Study the drawing (mm; zero at the part's minimum x, y, z) and answer. A direction names the side the tool comes from. Round coordinates to 2 decimals unless told otherwise and drop trailing zeros. Write each loop counter-clockwise with the first axis right and the second up, starting at its lowest first coordinate (ties: lowest second). Pieces come first, ordered by that corner, then holes. Notation, with made-up numbers: (17.25, 43.25) -> (51.25, 43.25) arc R19 cw to (51.25, 76.25) -> close; hole circle Ø7 at (71.25, 63.25). An arc over 180 degrees is marked (long way). Return JSON: item names as keys, results as strings.
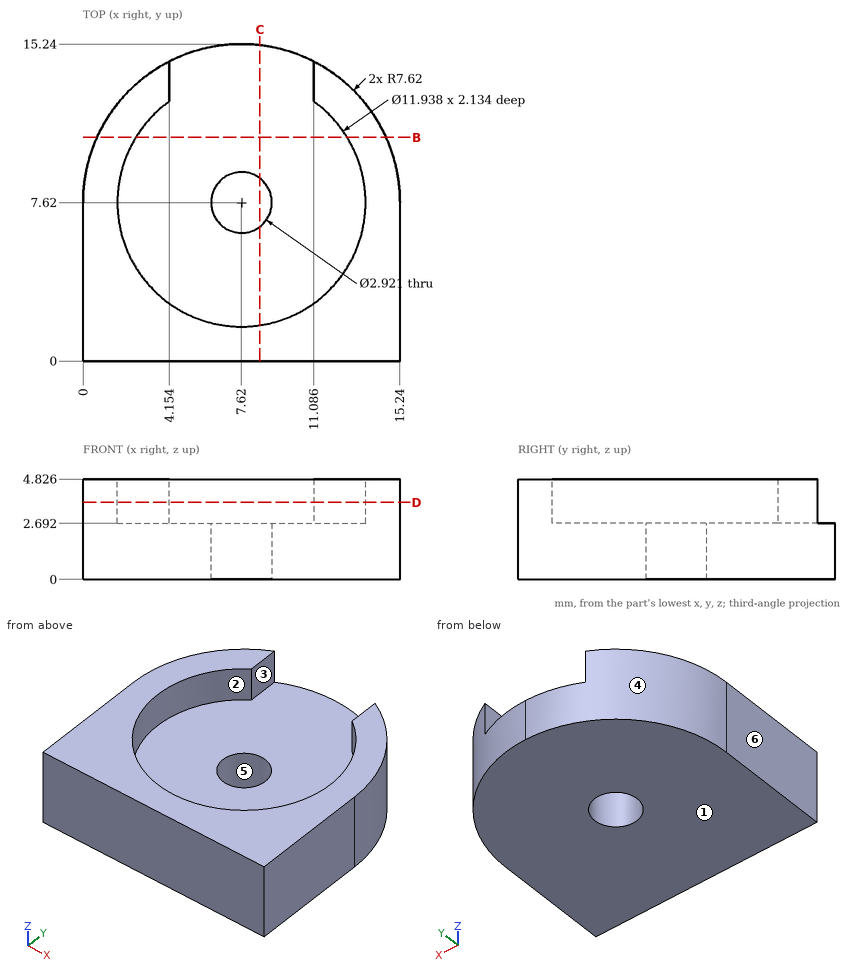
Item 1: Section B-B (y = 10.75) is taken. Give the vertices of the cut face in (x, z).
Worked answers:
{"outline": "(0.67, 0) -> (14.57, 0) -> (14.57, 4.83) -> (12.7, 4.83) -> (12.7, 2.69) -> (2.54, 2.69) -> (2.54, 4.83) -> (0.67, 4.83) -> close"}
Item 2: Flat-ended cylindrical pins translate along their axes: pin 1 (4 mm diameter, centred on x = 7.62, y = 7.62, fed in from -Z); pin 2 (1 mm diameter, centred on y = 13.5, z = 4, fed in from +X) (1 decimal); pin 3 (0.6 mm diameter, centred on y = 13.5, z = 3.5, fed in from -X). Find the tip coordinate at first contact, or state that the pin passes through.
Worked answers:
{"pin 1": "stops at z = 0", "pin 2": "stops at x = 13", "pin 3": "stops at x = 2.43"}
Item 3: For a pull along Y with two mould halves and no side action, classify the marked faces 4, 5 and 6 as released by +Y, released by -Y, zero draft, split by the parting line, or undercut.
Worked answers:
{"face 4": "released by +Y", "face 5": "undercut", "face 6": "zero draft"}
Item 4: A tool of negligible diameter and unlimited length cuts with its end or side. For the marked faces 1, 2 and 3, from which of +Z, -Z, +X, -X, +Y, -Y can it reach the whole face along a straight path? Write none if from no direction.
Worked answers:
{"face 1": "-Z, +X, -X, +Y, -Y", "face 2": "+Z", "face 3": "+Z, +Y"}
Item 5: Straight lines are drawn through the part: L1, parallel to Y at x = 7.62, z = 2.15; L2, parallel to X at y = 7.62, z = 4.05; L3, parallel to Z at x = 8, y = 13.5. For each, find the intervals that lie inside material, in ascending order. Write a range as [from, to].
Worked answers:
{"L1": "y = [0, 6.16], [9.08, 15.24]", "L2": "x = [0, 1.65], [13.59, 15.24]", "L3": "z = [0, 2.69]"}
Item 6: Section C-C (x = 8.5) is taken. Give the vertices of the cut face in (y, z) (1 decimal).
Worked answers:
{"outline": "(0, 0) -> (6.5, 0) -> (6.5, 2.7) -> (1.7, 2.7) -> (1.7, 4.8) -> (0, 4.8) -> close; (8.8, 0) -> (15.2, 0) -> (15.2, 2.7) -> (8.8, 2.7) -> close"}
Item 7: Section D-D (z = 3.7) is taken. Give the vertices of the cut face in (x, y) (1 decimal).
Worked answers:
{"outline": "(0, 0) -> (15.2, 0) -> (15.2, 7.6) arc R7.6 ccw to (11.1, 14.4) -> (11.1, 12.5) arc R6 cw (long way) to (4.2, 12.5) -> (4.2, 14.4) arc R7.6 ccw to (0, 7.6) -> close"}
